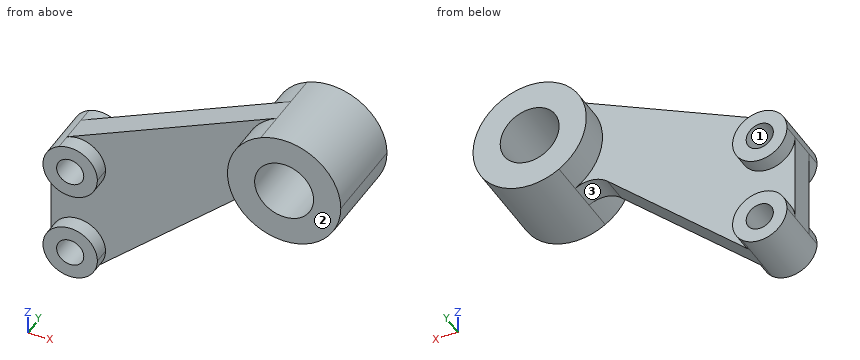
from build123d import *

# Parameters (mm, degrees)
F1_DEPTH = 5.9944
F0_R     = 13.0048
F2_DEPTH = 20.0025
F0_R_2   = 5.9944
F3_DEPTH = 13.0048


with BuildPart() as f1:
    # F0 (on Front) → F1 (new body, symmetric)
    with BuildSketch(Plane.XZ):
        with BuildLine():
            ThreePointArc((-12.949346, 32.124952), (-24.961282, 55.017041), (-10.294693, 76.306136))
            Line((-10.294693, 76.306136), (-102.934025, 34.457115))
            ThreePointArc((-102.934025, 34.457115), (-91.484026, 33.602816), (-85.9917, 23.519828))
            ThreePointArc((-85.9917, 23.519828), (-97.9932, 11.518328), (-109.9947, 23.519828))
            Line((-109.9947, 23.519828), (-109.9947, -16.485172))
            ThreePointArc((-109.9947, -16.485172), (-97.9932, -4.483672), (-85.9917, -16.485172))
            ThreePointArc((-85.9917, -16.485172), (-87.036779, -21.383422), (-89.990008, -25.428602))
            Line((-89.990008, -25.428602), (-27.152389, 30.802793))
            ThreePointArc((-27.152389, 30.802793), (-20.268898, 33.806017), (-12.949346, 32.124952))
        make_face()
    extrude(amount=F1_DEPTH, both=True)

    # F0 (on Front) → F2 (join, symmetric)
    with BuildSketch(Plane.XZ):
        with BuildLine():
            ThreePointArc((-12.949346, 32.124952), (12.278025, 31.732712), (25.0063, 53.517228))
            ThreePointArc((25.0063, 53.517228), (13.562501, 74.526121), (-10.294693, 76.306136))
            ThreePointArc((-10.294693, 76.306136), (-24.961282, 55.017041), (-12.949346, 32.124952))
        make_face()
        with Locations((0, 53.517228)):
            Circle(F0_R, mode=Mode.SUBTRACT)
    extrude(amount=F2_DEPTH, both=True)

    # F0 (on Front) → F3 (join, symmetric)
    with BuildSketch(Plane.XZ):
        with BuildLine():
            ThreePointArc((-85.9917, 23.519828), (-91.484026, 33.602816), (-102.934025, 34.457115))
            ThreePointArc((-102.934025, 34.457115), (-108.076189, 30.029001), (-109.9947, 23.519828))
            ThreePointArc((-109.9947, 23.519828), (-97.9932, 11.518328), (-85.9917, 23.519828))
        make_face()
        with Locations((-97.9932, 23.519828)):
            Circle(F0_R_2, mode=Mode.SUBTRACT)
        with BuildLine():
            ThreePointArc((-109.9947, -16.485172), (-102.89145, -27.441593), (-89.990008, -25.428602))
            ThreePointArc((-89.990008, -25.428602), (-87.036779, -21.383422), (-85.9917, -16.485172))
            ThreePointArc((-85.9917, -16.485172), (-97.9932, -4.483672), (-109.9947, -16.485172))
        make_face()
        with Locations((-97.9932, -16.485172)):
            Circle(F0_R_2, mode=Mode.SUBTRACT)
    extrude(amount=F3_DEPTH, both=True)


solid = f1.part
CAD build for the part. Positions are in the model's coordinates, mm. Face numbers are marked on the shaded views. Coordinates: 2 decimals unless noted, no trailing zeros. Loops run counter-clockwise (first coordinate to the right, second up) from the corner with the lowest first, then second, coordinate; pieces in that order, holes last. Notation, with made-up numbers: (25.5, 0.5) -> (53.5, 0.5) arc R22 cw to (53.5, 31.5) -> close; hole circle Ø8 at (64, 11.25). An arc over 180 degrees is marked (long way). One line per item, written item: value.
1. Pull direction Z, two halves, no side cores. Call the marked faces 1, 2 and 3: pulls with the +Z half, pulls with the -Z half, needs draft (parallel to the pull), parting line crosses it, or undercut.
Answers:
face 1: undercut
face 2: needs draft
face 3: pulls with the -Z half
2. Slice it at A-A on x = 0. Write the cut outline in (y, z), and give its area (3 significant figures).
Answers:
outline: (-20, 28.51) -> (20, 28.51) -> (20, 40.51) -> (-20, 40.51) -> close; (-20, 66.52) -> (20, 66.52) -> (20, 78.52) -> (-20, 78.52) -> close
area: 960 mm^2
3. Drill centre lines: line 1 (Z direction, x = 0, y = -4); line 2 (Z direction, x = -92.5, y = 5); line 3 (Y direction, x = -59, z = 7.5). Where is each one in solid material? Low to high. Write a range as [from, to].
Answers:
line 1: z = [28.51, 40.51], [66.52, 78.52]
line 2: z = [-27.16, -18.88], [-14.09, 21.12], [25.92, 39.17]
line 3: y = [-5.99, 5.99]
4. Slice it at C-C on z = -18. Write the cut outline in (x, y).
Answers:
outline: (-109.9, -13) -> (-103.79, -13) -> (-103.79, 13) -> (-109.9, 13) -> close; (-92.19, -13) -> (-86.09, -13) -> (-86.09, -5.99) -> (-81.69, -5.99) -> (-81.69, 5.99) -> (-86.09, 5.99) -> (-86.09, 13) -> (-92.19, 13) -> close
5. Slice it at B-B on y = -4.5. Write the cut outline in (x, z).
Answers:
outline: (-109.99, -16.49) arc R12 ccw to (-89.99, -25.43) -> (-27.15, 30.8) arc R11.99 cw to (-12.95, 32.12) arc R25.01 ccw (long way) to (-10.29, 76.31) -> (-102.93, 34.46) arc R12 ccw to (-109.99, 23.52) -> close; hole circle Ø11.99 at (-97.99, -16.49); hole circle Ø11.99 at (-97.99, 23.52); hole circle Ø26.01 at (0, 53.52)
6. Slice it at D-D on z = 47.5. Write the cut outline in (x, y).
Answers:
outline: (-74.06, -5.99) -> (-24.27, -5.99) -> (-24.27, -20) -> (-11.53, -20) -> (-11.53, 20) -> (-24.27, 20) -> (-24.27, 5.99) -> (-74.06, 5.99) -> close; (11.53, -20) -> (24.27, -20) -> (24.27, 20) -> (11.53, 20) -> close
7. Flat gauge pins, fed straight in: P1, Ø7, axis at x = -99.5, z = -11.5, coming from the +Y side; P2, Ø6, axis at y = -3.5, z = 46, coming from the +X side; P3, Ø10, axis at x = -89, y = 2.5, coming from the -Z side. Where does each tip first touch, or does it go through?
Answers:
P1: stops at y = 13
P2: stops at x = 24.59
P3: stops at z = -27.8
